Verification items for the finished model (mm, model axes). Face numbers are marked on the shaded views. A direction names the side the tool comes from. Coordinates: 2 decimals unless noted, no trailing zeros. Loops run counter-clockwise (first coordinate to the right, second up) from the corner with the lowest first, then second, coordinate; pieces in that order, holes last. Notation, with made-up numbers: (65.25, 3) -> (74.25, 3) arc R35 ccw to (74.25, 39) -> close; hole circle Ø9 at (78, 62.5). An arc over 180 degrees is marked (long way). Answer as a JSON object with one key per item and string values. Group by question number.
Q1. Cross-section at B-B on x = 4.75. Record the boundary of the cut face in (y, z).
Q2. Scan lines: L1, parallel to Y at x = 0, z = -7.1; L2, parallel to Z at x = 3.25, y = 65. Record each from-to range of solid material in increasing order.
Q3. Release check for a two-part mould opening along X. For the marked faces 3, 4 and 5 record: released by +X, released by -X, zero draft, split by the parting line, or undercut.
Q4. Cross-section at D-D on y = 95. Record the boundary of the cut face in (x, z).
Q5. Set-up check for the marked faces 1 and 2: record each of +Z, -Z, +X, -X, +Y, -Y from which the full face is reachable in a straight line by a thin tool's end or side.
Q6. Cross-section at C-C on z = 3.5. Record the boundary of the cut face in (x, y), and give its area (3 significant figures).
Q7. Cross-section at A-A on y = 25. Record the boundary of the cut face in (x, z), and give its area (3 significant figures).
```python
from build123d import *

# Parameters (mm, degrees)
SKETCH_1_W          = 15
SKETCH_1_H          = 15
SKETCH_1_W_2        = 13
SKETCH_1_H_2        = 13
EXTRUDE_1_DEPTH     = 120
SKETCH_2_R          = 1.5
CUT_EXTRUDE_1_DEPTH = 122.166208161
SKETCH_3_R          = 1.5
CUT_EXTRUDE_2_DEPTH = 122.166208161


with BuildPart() as part:
    # 草图1 → 凸台-拉伸1 (new body)
    with BuildSketch(Plane(origin=(0, 0, 0), x_dir=(1, 0, 0), z_dir=(0, 1, 0))):
        Rectangle(SKETCH_1_W, SKETCH_1_H)
        Rectangle(SKETCH_1_W_2, SKETCH_1_H_2, mode=Mode.SUBTRACT)
    extrude(amount=EXTRUDE_1_DEPTH)

    # 草图2 → 切除-拉伸1 (cut, through all)
    with BuildSketch(Plane.XY.offset(7.5)):
        with Locations((0, 104.5)):
            Circle(SKETCH_2_R)
        with Locations((0, 81.5)):
            Circle(SKETCH_2_R)
    extrude(amount=-CUT_EXTRUDE_1_DEPTH, mode=Mode.SUBTRACT)

    # 草图3 → 切除-拉伸2 (cut, through all)
    with BuildSketch(Plane.ZY.offset(7.5)):
        with Locations((0, 10)):
            Circle(SKETCH_3_R)
        with Locations((0, 25)):
            Circle(SKETCH_3_R)
        Polygon((-0.5, 0), (7.5, 0), (7.5, 8), align=None)
    extrude(amount=-CUT_EXTRUDE_2_DEPTH, mode=Mode.SUBTRACT)


solid = part.part
```
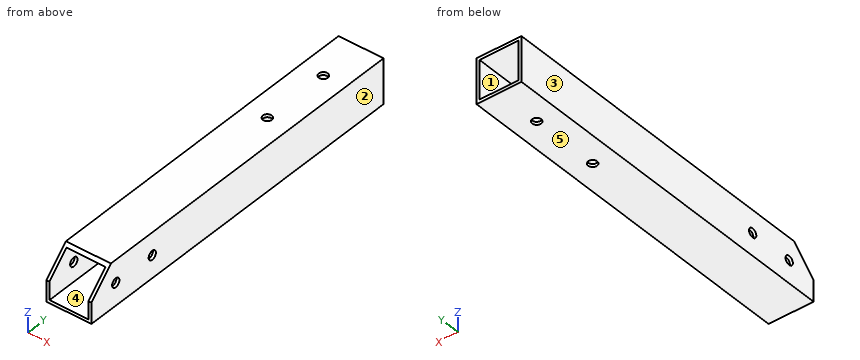
Computed values:
{
 "1": {"outline": "(0, -7.5) -> (120, -7.5) -> (120, -6.5) -> (0, -6.5) -> close; (7, 6.5) -> (120, 6.5) -> (120, 7.5) -> (8, 7.5) -> close"},
 "2": {"L1": "y = 0 to 80, 83 to 103, 106 to 120", "L2": "z = -7.5 to -6.5, 6.5 to 7.5"},
 "3": {"face 3": "released by -X", "face 4": "undercut", "face 5": "zero draft"},
 "4": {"outline": "(-7.5, -7.5) -> (7.5, -7.5) -> (7.5, 7.5) -> (-7.5, 7.5) -> close; hole (-6.5, -6.5) -> (6.5, -6.5) -> (6.5, 6.5) -> (-6.5, 6.5) -> close"},
 "5": {"face 1": "+Y, -Y", "face 2": "+Z, -Z, +X, +Y, -Y"},
 "6": {"outline": "(-7.5, 4) -> (-6.5, 4) -> (-6.5, 120) -> (-7.5, 120) -> close; (6.5, 4) -> (7.5, 4) -> (7.5, 120) -> (6.5, 120) -> close", "area": "232 mm²"},
 "7": {"outline": "(-7.5, -7.5) -> (7.5, -7.5) -> (7.5, -1.5) -> (6.5, -1.5) -> (6.5, -6.5) -> (-6.5, -6.5) -> (-6.5, -1.5) -> (-7.5, -1.5) -> close; (-7.5, 1.5) -> (-6.5, 1.5) -> (-6.5, 6.5) -> (6.5, 6.5) -> (6.5, 1.5) -> (7.5, 1.5) -> (7.5, 7.5) -> (-7.5, 7.5) -> close", "area": "50.0 mm²"}
}
